Here's how the part is built. I have some questions about the finished solid (model axes, mm). A direction names the side the tool comes from. Round coordinates to 2 decimals unless told otherwise and drop trailing zeros. Write each loop counter-clockwise with the first axis right and the second up, starting at its lowest first coordinate (ties: lowest second). Pieces come first, ordered by that corner, then holes. Notation, with made-up numbers: (4.5, -1) - (58.5, -1) arc R13 cw to (58.5, 13) - close; hole circle Ø4 at (-24.75, 31). An arc over 180 degrees is marked (long way). One line per question, with ' | ' between items. Start each with the question number.
(1) Will this pin go through, and if not, where does the flat tip stop? pin 1 (3 mm diameter, centred on y = -16, z = 12.5, fed in from -X).
(2) Imagine slicing it at B-B (z = 10.5). Write out the boundary of the cut face in (x, y).
(3) Imagine slicing it at A-A (x = 10.25). Write out the boundary of the cut face in (y, z).
(4) If I drill on L1, parallel to Z at x = 14.75, y = -24; L2, parallel to Y at x = 13.5, z = 6; L3, parallel to Y at x = 8.5, z = 13.5, over which ranges is the centre line in solid material (lowest first)?
(5) Imagine slicing it at C-C (y = -11.5). Write out the boundary of the cut face in (x, z).
(6) Thinking about a two-plate mould opening in Z: for faces 3 (the flat face through (9, -15, 0)), 4 (the cylindrical face through (9.367, -0.485, 14.489)), 5 (the flat face through (9, -15, 12)), which applies, pulls with the +Z half, pulls with the -Z half, needs draft (parallel to the pull), parting line crosses it, or undercut?
(7) For faces 1 (the flat face through (19, -15.2, 2.6)), 2 (the flat face through (9, -3, 7)), which set-ups out of +Z, -Z, +X, -X, +Y, -Y let a thin tool reach every point of the face, with its end or its side?
from build123d import *

# Parameters (mm, degrees)
F0_W     = 24
F0_H     = 9
F1_DEPTH = 19


with BuildPart() as f1:
    # F0 (on Right) → F1 (new body)
    with BuildSketch(Plane.YZ):
        with BuildLine():
            Line((-30, 0), (0, 0))
            Line((0, 0), (0, 13.3))
            ThreePointArc((0, 13.3), (-0.497918, 14.502082), (-1.7, 15))
            Line((-1.7, 15), (-13.862342, 15))
            Line((-13.862342, 15), (-28.3, 15))
            ThreePointArc((-28.3, 15), (-29.502082, 14.502082), (-30, 13.3))
            Line((-30, 13.3), (-30, 0))
        make_face()
        with Locations((-15, 7.5)):
            Rectangle(F0_W, F0_H, mode=Mode.SUBTRACT)
    extrude(amount=F1_DEPTH)


solid = f1.part
Check sheet entries:
1) pin 1: x = 0
2) outline: (0, -30) - (19, -30) - (19, -27) - (0, -27) - close; (0, -3) - (19, -3) - (19, 0) - (0, 0) - close
3) outline: (-30, 0) - (0, 0) - (0, 13.3) arc R1.7 ccw to (-1.7, 15) - (-28.3, 15) arc R1.7 ccw to (-30, 13.3) - close; hole (-27, 3) - (-3, 3) - (-3, 12) - (-27, 12) - close
4) L1: 0 to 3, 12 to 15 | L2: -30 to -27, -3 to 0 | L3: -29.99 to -0.01
5) outline: (0, 0) - (19, 0) - (19, 3) - (0, 3) - close; (0, 12) - (19, 12) - (19, 15) - (0, 15) - close
6) face 3: pulls with the -Z half | face 4: pulls with the +Z half | face 5: undercut
7) face 1: +Z, -Z, +X, +Y, -Y | face 2: +X, -X
